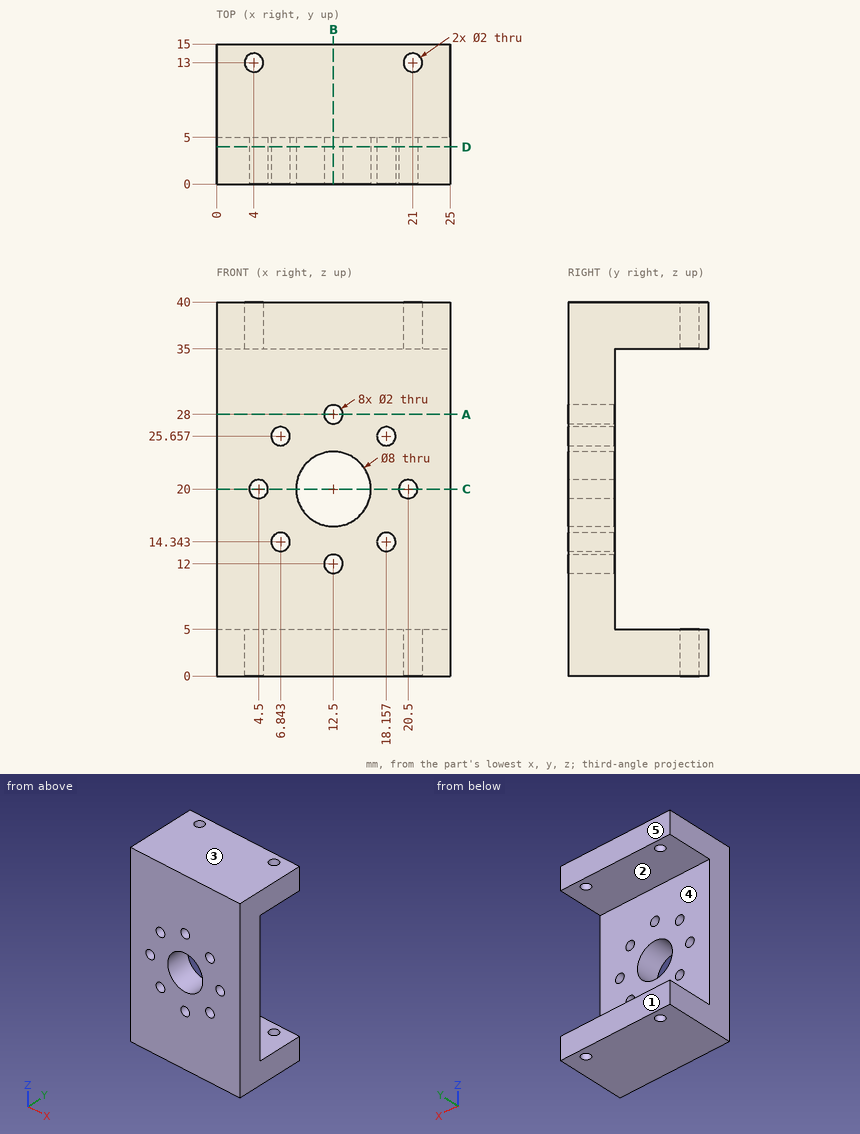
Could you check a few things on this drawing? It's one solid part, dimensions in mm from its lowest x, y, z. A direction names the side the tool comes from. Round coordinates to 2 decimals unless told otherwise and drop trailing zeros. Order: outer loops, then holes, each group sorted by start corner. A loop starts at its lowest first (then second) coordinate and runs counter-clockwise, first axis right, second up. Notation, with made-up numbers: M 35.25,49 L 62.25,49 A6 cw 62.25,54 Z; hole C -39.75,61.25 d2. An arc over 180 degrees is marked long. One line per item, written item: value.
(1) Imagine slicing it at C-C (z = 20). Write out the boundary of the cut face in (x, y), and give its area (3 significant figures).
Ans:
outline: M 0,0 L 3.5,0 L 3.5,5 L 0,5 Z; M 5.5,0 L 8.5,0 L 8.5,5 L 5.5,5 Z; M 16.5,0 L 19.5,0 L 19.5,5 L 16.5,5 Z; M 21.5,0 L 25,0 L 25,5 L 21.5,5 Z
area: 65.0 mm^2
(2) Which directions (+Z, -Z, +X, -X, +Y, -Y) give clear straight access to the entire face, cutting with the end or side of a thin tool? Please do the marked faces 4 and 5.
Ans:
face 4: +X, -X, +Y
face 5: +Z, -Z, +X, -X, +Y
(3) I'm going to push flat-ended pins straight in: P1, Ø2.5, axis at x = 6.84, z = 25.66, coming from the +Y side; P2, Ø1.2, axis at x = 12.5, z = 28, coming from the -Y side; P3, Ø13, axis at x = 12.5, z = 20, coming from the -Y side. Where does each tip first touch, or does it pass through?
Ans:
P1: stops at y = 5
P2: passes through
P3: stops at y = 0
(4) If we mould it in two halves opening along Z, with no side actions, what happens to the marked faces 1, 2 and 3? For each: released by +Z, released by -Z, zero draft, split by the parting line, or undercut.
Ans:
face 1: zero draft
face 2: undercut
face 3: released by +Z
(5) I need wall thicknesses on line 1 along X through (y, z) = (1.1, 20); line 2 along Z through (x, y) = (13, 6.25); line 3 along Y through (x, z) = (4, 38.5). Which ranges of each line are inside material? Lowest first, please. Write a range as from..to.
Ans:
line 1: x = 0..3.5, 5.5..8.5, 16.5..19.5, 21.5..25
line 2: z = 0..5, 35..40
line 3: y = 0..12, 14..15
(6) Imagine slicing it at B-B (x = 12.5). Write out the boundary of the cut face in (y, z), and give its area (3 significant figures).
Ans:
outline: M 0,0 L 15,0 L 15,5 L 5,5 L 5,11 L 0,11 Z; M 0,13 L 5,13 L 5,16 L 0,16 Z; M 0,24 L 5,24 L 5,27 L 0,27 Z; M 0,29 L 5,29 L 5,35 L 15,35 L 15,40 L 0,40 Z
area: 240 mm^2
(7) Imagine slicing it at A-A (z = 28). Write out the boundary of the cut face in (x, y).
Ans:
outline: M 0,0 L 11.5,0 L 11.5,5 L 0,5 Z; M 13.5,0 L 25,0 L 25,5 L 13.5,5 Z
(8) Imagine slicing it at D-D (y = 4). Count the separate pieces of the cut face and the enclosed holes in it, and give its area (3 significant figures).
Ans:
separate pieces: 1
enclosed holes: 9
area: 925 mm^2
